For this review, take the finished solid that the model builds, in its own axes (mm). A direction names the side the tool comes from. Give positions to 0.01 mm unless a question says otherwise; leave off trailing zeros. Write each loop counter-clockwise with the first axis right and the second up, starting at its lowest first coordinate (ties: lowest second). Pieces come first, ordered by that corner, then holes.
1) We need section B-B on y = 0.5. Give the number of separate pieces and of enclosed holes in the cut face, and give its area (3 significant figures).
2) Machinability: for faces 1 (the face through (19.604, 3.873, -1.277)), 2 (the face through (16, 0, 0)), which of the approach directions +Z, -Z, +X, -X, +Y, -Y give a long, thin tool a straight path to every point of the face, cutting with its end or side? Answer none if there is none.
3) Draft analysis for pull direction Z (two halves, no side actions). For faces 3 (the face through (-4.25, 0.99, 0.09)), 4 (the face through (24.955, 0.986, 0.456)), 5 (the face through (28, 2, -1)), state which applies: pulls with the +Z half, pulls with the -Z half, needs draft (parallel to the pull), parting line crosses it, or undercut.
4) We need section D-D on z = -2.25. Give the boundary of the cut face in (x, y).
5) We need section A-A on x = 23.05. Give the boundary of the cut face in (y, z).
6) Wall thickness on line 1 along Z through (x, y) = (3.05, 0.5); line 2 along X through (y, z) = (4.75, 0); line 3 along Y through (x, z) = (21.5, -1.75): over which ranges is each line inside the solid? List them lowest first.
7) For P1, Ø2.5, axis at x = 23.05, z = 0, coming from the -Y side; P2, Ø3, axis at x = 16.5, z = 1, coming from the +Y side; P3, Ø1.5, axis at y = 2, z = -3, coming from the -X side; P4, Ø1, axis at y = 4.5, z = 1, coming from the -X side, all flat-tipped, find the tip position at first contact; note any pin that passes through.
from build123d import *

# Parameters (mm, degrees)
SKETCH_1_R          = 0.75
EXTRUDE_1_DEPTH     = 2
SKETCH_2_R          = 4.25
EXTRUDE_2_DEPTH     = 3.8
SKETCH_3_R          = 3
CUT_EXTRUDE_1_DEPTH = 3.8


with BuildPart() as part:
    # Эскиз1 → Бобышка-Вытянуть1 (new body)
    with BuildSketch(Plane(origin=(0, 0, 0), x_dir=(1, 0, 0), z_dir=(0, 1, 0))):
        with BuildLine():
            Line((0, 4.25), (31.1, 4.25))
            ThreePointArc((31.1, 4.25), (35.35, 0), (31.1, -4.25))
            Line((31.1, -4.25), (0, -4.25))
            ThreePointArc((0, -4.25), (-4.25, 0), (0, 4.25))
        make_face()
        with Locations((8.05, 0)):
            Circle(SKETCH_1_R, mode=Mode.SUBTRACT)
        with Locations((23.05, 0)):
            Circle(SKETCH_1_R, mode=Mode.SUBTRACT)
        with Locations((25.55, 0)):
            Circle(SKETCH_1_R, mode=Mode.SUBTRACT)
        with Locations((28.05, 0)):
            Circle(SKETCH_1_R, mode=Mode.SUBTRACT)
        with Locations((30.55, 0)):
            Circle(SKETCH_1_R, mode=Mode.SUBTRACT)
        with Locations((5.55, 0)):
            Circle(SKETCH_1_R, mode=Mode.SUBTRACT)
        with Locations((3.05, 0)):
            Circle(SKETCH_1_R, mode=Mode.SUBTRACT)
        with Locations((0.55, 0)):
            Circle(SKETCH_1_R, mode=Mode.SUBTRACT)
    extrude(amount=EXTRUDE_1_DEPTH)

    # Эскиз2 → Бобышка-Вытянуть2 (add)
    with BuildSketch(Plane(origin=(0, 2, 0), x_dir=(1, 0, 0), z_dir=(0, 1, 0))):
        with Locations((15.55, 0)):
            Circle(SKETCH_2_R)
    extrude(amount=EXTRUDE_2_DEPTH)

    # Эскиз3 → Вырез-Вытянуть1 (cut)
    with BuildSketch(Plane(origin=(0, 5.8, 0), x_dir=(1, 0, 0), z_dir=(0, 1, 0))):
        with Locations((15.55, 0)):
            Circle(SKETCH_3_R)
    extrude(amount=-CUT_EXTRUDE_1_DEPTH, mode=Mode.SUBTRACT)


solid = part.part
Results list:
1. separate pieces: 1
1. enclosed holes: 8
1. area: 307 mm2
2. face 1: +Y
2. face 2: +Z, -Z, +X, -X, -Y
3. face 3: parting line crosses it
3. face 4: undercut
3. face 5: needs draft
4. outline: (-3.61, 0) - (34.71, 0) - (34.71, 2) - (19.16, 2) - (19.16, 5.8) - (17.53, 5.8) - (17.53, 2) - (13.57, 2) - (13.57, 5.8) - (11.94, 5.8) - (11.94, 2) - (-3.61, 2) - close
5. outline: (0, -4.25) - (2, -4.25) - (2, -0.75) - (0, -0.75) - close; (0, 0.75) - (2, 0.75) - (2, 4.25) - (0, 4.25) - close
6. line 1: z = -4.25 to -0.75, 0.75 to 4.25
6. line 2: x = 11.3 to 12.55, 18.55 to 19.8
6. line 3: y = 0 to 2
7. P1: stops at y = 0
7. P2: stops at y = 2
7. P3: stops at x = -3.61
7. P4: stops at x = 11.33
